Here's how the part is built. I have some questions about the finished solid (model axes, mm). Face numbers are marked on the shaded views. A direction names the side the tool comes from. Give positions to 0.01 mm unless a question says otherwise; leave off trailing zeros. Loops run counter-clockwise (first coordinate to the right, second up) from the corner with the lowest first, then second, coordinate; pieces in that order, holes last. Notation, with made-up numbers: (78.5, 84.25) - (91.5, 84.25) arc R26 cw to (91.5, 114.25) - close; hole circle Ø1 at (-36.5, 57.5). An arc over 180 degrees is marked (long way). Put each result on its own line as item: value. Start each with the question number.
from build123d import *

# Parameters (mm, degrees)
SKETCH1_R           = 2.2
BOSS_EXTRUDE1_DEPTH = 100
SKETCH5_W           = 15
SKETCH5_H           = 15
SKETCH5_R           = 2.2
CUT_EXTRUDE2_DEPTH  = 91
CUT_EXTRUDE3_DEPTH  = 112.803398875
LPATTERN1_COUNT     = 2
LPATTERN1_PITCH     = 35
CUT_EXTRUDE4_DEPTH  = 5
CHAMFER1_SIZE       = 2.5


with BuildPart() as part:
    # Sketch1 → Boss-Extrude1 (new body)
    with BuildSketch(Plane.XY):
        Polygon((-25, 22.5), (-25, 7.5), (-40, 7.5), (-40, -7.5), (40, -7.5), (40, 7.5), (25, 7.5), (25, 22.5), (10, 22.5), (10, 7.5), (-10, 7.5), (-10, 22.5), align=None)
        with Locations((-17.5, 15)):
            Circle(SKETCH1_R, mode=Mode.SUBTRACT)
        with Locations((-32.5, 0)):
            Circle(SKETCH1_R, mode=Mode.SUBTRACT)
        with Locations((17.5, 15)):
            Circle(SKETCH1_R, mode=Mode.SUBTRACT)
        with Locations((32.5, 0)):
            Circle(SKETCH1_R, mode=Mode.SUBTRACT)
    extrude(amount=BOSS_EXTRUDE1_DEPTH)

    # Sketch5 → Cut-Extrude2 (cut)
    # profile 1 of 4: a face of its own
    with BuildSketch(Plane(origin=(0, 0, 0), x_dir=(-1, 0, 0), z_dir=(0, 0, -1))):
        with Locations((-32.5, 0)):
            Rectangle(SKETCH5_W, SKETCH5_H)
        with Locations(Location((-32.5, 0, 0), (0, 0, 180))):
            Circle(SKETCH5_R, mode=Mode.SUBTRACT)
    # profile 2 of 4: a face of its own
    with BuildSketch(Plane(origin=(0, 0, 0), x_dir=(-1, 0, 0), z_dir=(0, 0, -1))):
        with Locations((-17.5, 15)):
            Rectangle(SKETCH5_W, SKETCH5_H)
        with Locations(Location((-17.5, 15, 0), (0, 0, 180))):
            Circle(SKETCH5_R, mode=Mode.SUBTRACT)
    # profile 3 of 4: a face of its own
    with BuildSketch(Plane(origin=(0, 0, 0), x_dir=(-1, 0, 0), z_dir=(0, 0, -1))):
        with Locations((17.5, 15)):
            Rectangle(SKETCH5_W, SKETCH5_H)
        with Locations(Location((17.5, 15, 0), (0, 0, 180))):
            Circle(SKETCH5_R, mode=Mode.SUBTRACT)
    # profile 4 of 4: a face of its own
    with BuildSketch(Plane(origin=(0, 0, 0), x_dir=(-1, 0, 0), z_dir=(0, 0, -1))):
        with Locations((32.5, 0)):
            Rectangle(SKETCH5_W, SKETCH5_H)
        with Locations(Location((32.5, 0, 0), (0, 0, 180))):
            Circle(SKETCH5_R, mode=Mode.SUBTRACT)
    extrude(amount=-CUT_EXTRUDE2_DEPTH, mode=Mode.SUBTRACT)

    # Sketch6 → Cut-Extrude3 (cut, through all)
    with BuildSketch(Plane.XZ.offset(7.5)):
        with BuildLine():
            Line((5, 70.5), (5, 20.5))
            ThreePointArc((5, 20.5), (0, 15.5), (-5, 20.5))
            Line((-5, 20.5), (-5, 70.5))
            ThreePointArc((-5, 70.5), (0, 75.5), (5, 70.5))
        make_face()
        with BuildLine():
            Line((-11.9, 80.5), (-11.9, 10.5))
            ThreePointArc((-11.9, 10.5), (-14, 8.4), (-16.1, 10.5))
            Line((-16.1, 10.5), (-16.1, 80.5))
            ThreePointArc((-16.1, 80.5), (-14, 82.6), (-11.9, 80.5))
        make_face()
        with BuildLine():
            Line((11.9, 80.5), (11.9, 10.5))
            ThreePointArc((11.9, 10.5), (14, 8.4), (16.1, 10.5))
            Line((16.1, 10.5), (16.1, 80.5))
            ThreePointArc((16.1, 80.5), (14, 82.6), (11.9, 80.5))
        make_face()
    extrude(amount=-CUT_EXTRUDE3_DEPTH, mode=Mode.SUBTRACT)

    # Sketch2 → Cut-Revolve1 (revolve, cut)
    with BuildSketch(Plane(origin=(0, 15, 0), x_dir=(1, 0, 0), z_dir=(0, 1, 0)), mode=Mode.PRIVATE) as cut_revolve1_sk:
        Polygon((-17.5, -91), (-17.5, -94), (-15.3, -94), (-12.692139787, -91), align=None)
    cut_revolve1 = revolve(cut_revolve1_sk.sketch.rotate(Axis((-17.5, 15, 91), (0, 0, 1)), 180), axis=Axis((-17.5, 15, 91), (0, 0, 1)), mode=Mode.SUBTRACT)

    # LPattern1: Cut-Revolve1 ×2
    with Locations(*[(i * LPATTERN1_PITCH, 0, 0) for i in range(1, LPATTERN1_COUNT)]):
        add(cut_revolve1, mode=Mode.SUBTRACT)

    # Sketch8 → Cut-Revolve2 (revolve, cut)
    with BuildSketch(Plane.ZY.offset(32.5)):
        Polygon((91, 0), (94, 0), (94, 2.2), (91, 4.807860213), align=None)
    cut_revolve2 = revolve(axis=Axis((-32.5, 0, 91), (0, 0, 1)), mode=Mode.SUBTRACT)

    # Mirror3: Cut-Revolve2 across plane
    add(cut_revolve2.mirror(Plane(origin=(0, 0, 0), x_dir=(0, 0, 1), z_dir=(1, 0, 0))), mode=Mode.SUBTRACT)

    # Sketch7 → Cut-Extrude4 (cut)
    with BuildSketch(Plane(origin=(0, 7.5, 0), x_dir=(1, 0, 0), z_dir=(0, 1, 0))):
        with BuildLine():
            Line((-10.35, -10.5), (-10.35, -80.5))
            ThreePointArc((-10.35, -80.5), (-14, -84.15), (-17.65, -80.5))
            Line((-17.65, -80.5), (-17.65, -10.5))
            ThreePointArc((-17.65, -10.5), (-14, -6.85), (-10.35, -10.5))
        make_face()
        with BuildLine():
            Line((10.35, -10.5), (10.35, -80.5))
            ThreePointArc((10.35, -80.5), (14, -84.15), (17.65, -80.5))
            Line((17.65, -80.5), (17.65, -10.5))
            ThreePointArc((17.65, -10.5), (14, -6.85), (10.35, -10.5))
        make_face()
    extrude(amount=-CUT_EXTRUDE4_DEPTH, mode=Mode.SUBTRACT)

    # Chamfer1
    chamfer1_edges = [part.edges().sort_by_distance(p)[0] for p in [
        (-25, 0, 0),
        (25, 0, 0),
        (-25, 22.5, 95.5),
        (-10, 22.5, 95.5),
        (-10, 7.5, 95.5),
        (10, 7.5, 95.5),
        (10, 22.5, 95.5),
        (25, 22.5, 95.5),
        (40, 7.5, 95.5),
        (40, -7.5, 95.5),
        (-40, -7.5, 95.5),
        (-40, 7.5, 95.5),
    ]]
    chamfer(chamfer1_edges, length=CHAMFER1_SIZE)


solid = part.part
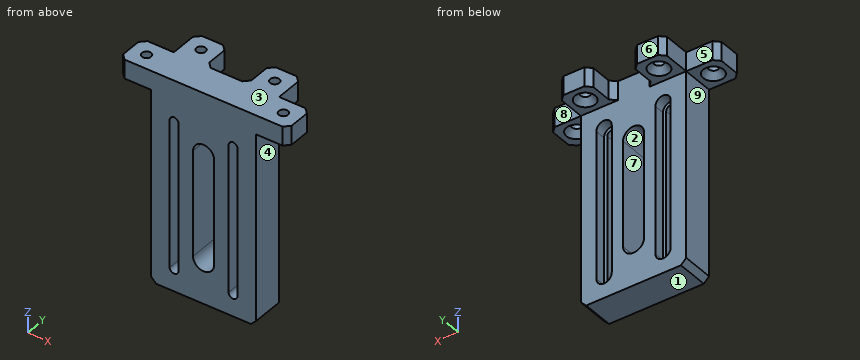
1) Suppose I cut it at B-B on z = 47. Please give me the cut outline in (x, y).
2) Thinking about a two-plate mould opening in Z: for the marked faces 1, 2, 3 and 4, which applies, pulls with the +Z half, pulls with the -Z half, needs draft (parallel to the pull), parting line crosses it, or undercut?
3) I'm going to push flat-ended pins straight in: P1, Ø2.5, axis at y = 5, z = 36.5, coming from the -X side; P2, Ø12, axis at y = 2, z = 45, coming from the +X side; P3, Ø7, axis at x = -17.5, y = 15, coming from the +Z side; P4, Ø1, axis at x = 18.5, z = 64, coming from the +Y side. Where does each tip first touch, or does it pass through?
4) Suppose I cut it at A-A on x = 0. Please give me the cut outline in (y, z), plus the area to 3 significant figures.
5) Which directions (+Z, -Z, +X, -X, +Y, -Y) give clear straight access to the entire face, cutting with the end or side of a thin tool? Please do the marked faces 5, 6, 7, 8 and 9.
6) I need wall thicknesses on line 1 (X direction, y = 15, z = 96.45); line 2 (X direction, y = 0, z = 98.25); line 3 (X direction, y = 4, z = 78). Which ranges of each line are inside material? Lowest first, please.
Ans:
1. outline: (-25, -7.5) - (-16.1, -7.5) - (-16.1, 2.5) - (-17.65, 2.5) - (-17.65, 7.5) - (-25, 7.5) - close; (-11.9, -7.5) - (-5, -7.5) - (-5, 7.5) - (-10.35, 7.5) - (-10.35, 2.5) - (-11.9, 2.5) - close; (5, -7.5) - (11.9, -7.5) - (11.9, 2.5) - (10.35, 2.5) - (10.35, 7.5) - (5, 7.5) - close; (16.1, -7.5) - (25, -7.5) - (25, 7.5) - (17.65, 7.5) - (17.65, 2.5) - (16.1, 2.5) - close
2. face 1: pulls with the -Z half
2. face 2: undercut
2. face 3: pulls with the +Z half
2. face 4: needs draft
3. P1: stops at x = -25
3. P2: stops at x = 25
3. P3: stops at z = 100
3. P4: stops at y = 7.5
4. outline: (-7.5, 0) - (7.5, 0) - (7.5, 15.5) - (-7.5, 15.5) - close; (-7.5, 75.5) - (7.5, 75.5) - (7.5, 100) - (-7.5, 100) - close
4. area: 600 mm²
5. face 5: +Z, -Z, -X, +Y
5. face 6: +Z, -Z, +X, -X, +Y
5. face 7: +Y, -Y
5. face 8: +Z, -Z, +X, +Y
5. face 9: -Z, -X, +Y, -Y
6. line 1: x = -25 to -19.7, -15.3 to -10, 10 to 15.3, 19.7 to 25
6. line 2: x = -40 to -34.7, -30.3 to 30.3, 34.7 to 40
6. line 3: x = -25 to -17.65, -10.35 to 10.35, 17.65 to 25
